For this review, take the finished solid that the model builds, in its own axes (mm). Face numbers are marked on the shaded views. A direction names the side the tool comes from. Round coordinates to 2 decimals unless told otherwise and drop trailing zeros. Order: outer loops, then holes, each group sorted by start corner. A loop starts at its lowest first (then second) coordinate and runs counter-clockwise, first axis right, second up. Notation, with made-up numbers: (57, -17) -> (78, -17) arc R25 ccw to (78, 22) -> close; hole circle Ø1 at (5.25, -11). An arc over 180 degrees is marked (long way). Use a Markdown table: item, result. Add a question column.
1) Draft analysis for pull direction Z (two halves, no side actions). For the marked faces 1, 2, 3 and 4, state which applies: pulls with the +Z half, pulls with the -Z half, needs draft (parallel to the pull), parting line crosses it, or undercut.
2) Consider section A-A (y = 0). State the section outline as (x, z) points (3 decimals).
3) Clearance check with flat-ended pins moving along their axes: P1, Ø4.5, axis at x = -0.5, y = -1, coming from the -Z side; P2, Ø3, axis at x = -4, y = 1.5, coming from the +Z side; P3, Ø0.7, axis at y = 8, z = -2.5, coming from the +X side. State where each tip first meets the part, or that it passes through.
4) Consider section C-C (z = -7.5). State the section outline as (x, y) points.
5) Consider section B-B (x = 6.75). State the section outline as (y, z) points, plus the area to 3 significant figures.
6) Machinability: for the marked faces 5, 6 and 7, which of the approach directions +Z, -Z, +X, -X, +Y, -Y give a long, thin tool a straight path to every point of the face, cutting with its end or side? Answer none if there is none.
7) Wall thickness on line 1 along Z through (x, y) = (-0.75, -6); line 2 along Y through (x, z) = (0, -26.05); line 3 along X through (y, z) = (12.75, 6.5): over which ranges is each line inside the solid? List them lowest first. Write a range as [from, to].
8) Consider section D-D (x = 0). State the section outline as (y, z) points (3 decimals), plus the area to 3 significant figures.
```python
from build123d import *

# Parameters (mm, degrees)
CROQUIS1_R              = 7.705
SALIENTE_EXTRUIR1_DEPTH = 4.35
SALIENTE_EXTRUIR2_START = -13.5
SALIENTE_EXTRUIR2_DEPTH = 18.5
SALIENTE_EXTRUIR3_DEPTH = 13.5
CROQUIS5_R              = 1.042712332
CORTAR_EXTRUIR1_DEPTH   = 2.5


with BuildPart() as part:
    # Croquis1 → Saliente-Extruir1 (new, symmetric)
    with BuildSketch(Plane.XY):
        Circle(CROQUIS1_R)
    saliente_extruir1 = extrude(amount=SALIENTE_EXTRUIR1_DEPTH, both=True)



with BuildPart() as body_2:
    # Croquis3 → Saliente-Extruir2 (new body)
    with BuildSketch(Plane.XY.offset(4.35).offset(SALIENTE_EXTRUIR2_START)):
        with BuildLine():
            Line((2, 8.034909184), (1.02204697, 8.135386739))
            ThreePointArc((1.02204697, 8.135386739), (0, 8.18775285), (-1.02204697, 8.135386739))
            Line((-1.02204697, 8.135386739), (-2, 8.034909184))
            Line((-2, 8.034909184), (-3.200003677, 11.21841322))
            ThreePointArc((-3.200003677, 11.21841322), (-3.248411026, 11.748541167), (-3.017934695, 12.228394865))
            Line((-3.017934695, 12.228394865), (-2.568482545, 12.743765532))
            ThreePointArc((-2.568482545, 12.743765532), (-2.445625709, 12.919659287), (-2.363117092, 13.117711661))
            Line((-2.363117092, 13.117711661), (-2, 14.346858197))
            Line((-2, 14.346858197), (2, 14.346858197))
            Line((2, 14.346858197), (2.363117092, 13.117711661))
            ThreePointArc((2.363117092, 13.117711661), (2.445625709, 12.919659287), (2.568482545, 12.743765532))
            Line((2.568482545, 12.743765532), (3.017934695, 12.228394865))
            ThreePointArc((3.017934695, 12.228394865), (3.248411026, 11.748541167), (3.200003677, 11.21841322))
            Line((3.200003677, 11.21841322), (2, 8.034909184))
        make_face()
    saliente_extruir2 = extrude(amount=SALIENTE_EXTRUIR2_DEPTH)


with BuildPart() as part_1:
    add(part.part)

    add(body_2.part)  # Saliente-Extruir3 merges body 2
    # Croquis4 → Saliente-Extruir3 (add)
    with BuildSketch(Plane.XY.offset(4.35)):
        with BuildLine():
            Line((1.529777798, 7.551609424), (1.529777798, 8.083221093))
            ThreePointArc((1.529777798, 8.083221093), (0, 8.18775285), (-1.529777798, 8.083221093))
            Line((-1.529777798, 8.083221093), (-1.529777798, 7.551609424))
            Line((-1.529777798, 7.551609424), (-1.529777798, 7.414435005))
            ThreePointArc((-1.529777798, 7.414435005), (0, 7.562302456), (1.529777798, 7.414435005))
            Line((1.529777798, 7.414435005), (1.529777798, 7.551609424))
        make_face()
    saliente_extruir3 = extrude(amount=-SALIENTE_EXTRUIR3_DEPTH)

    # Simetría2: Saliente-Extruir2, Saliente-Extruir3 across plane
    add(saliente_extruir2.mirror(Plane.XY.offset(-8.65)))
    add(saliente_extruir3.mirror(Plane.XY.offset(-8.65)))

    # Simetría3: Saliente-Extruir1 across plane
    add(saliente_extruir1.mirror(Plane.XY.offset(-8.65)))

    # Croquis5 → Cortar-Extruir1 (cut)
    with BuildSketch(Plane.XY.offset(9.35)):
        with Locations((0, 11.126169976)):
            Circle(CROQUIS5_R)
    cortar_extruir1 = extrude(amount=-CORTAR_EXTRUIR1_DEPTH, mode=Mode.SUBTRACT)

    # Simetría4: Cortar-Extruir1 across plane
    add(cortar_extruir1.mirror(Plane.XY.offset(-8.65)), mode=Mode.SUBTRACT)


solid = part_1.part
```
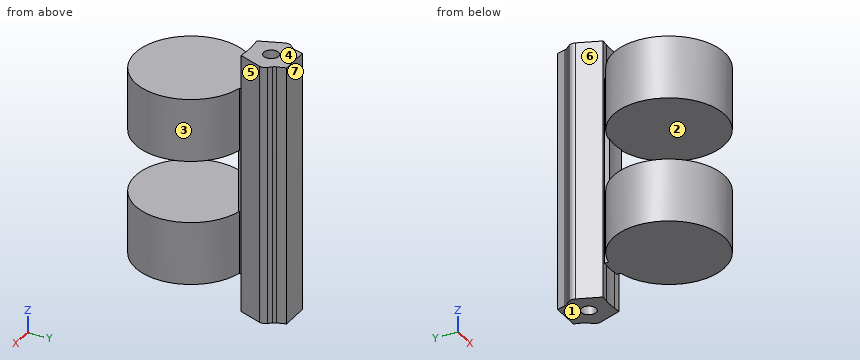
Results list:
| question | item | result |
|---|---|---|
| 1 | face 1 | pulls with the -Z half |
| 1 | face 2 | undercut |
| 1 | face 3 | needs draft |
| 1 | face 4 | pulls with the +Z half |
| 2 | outline | (-7.705, -21.65) -> (7.705, -21.65) -> (7.705, -12.95) -> (-7.705, -12.95) -> close; (-7.705, -4.35) -> (7.705, -4.35) -> (7.705, 4.35) -> (-7.705, 4.35) -> close |
| 3 | P1 | z = -21.65 |
| 3 | P2 | z = 4.35 |
| 3 | P3 | x = 2.12 |
| 4 | outline | (-3.2, 11.22) -> (-2, 8.03) -> (-1.53, 8.08) -> (-1.53, 7.41) arc R7.99 cw to (1.53, 7.41) -> (1.53, 8.08) -> (2, 8.03) -> (3.2, 11.22) arc R1 ccw to (3.02, 12.23) -> (2.57, 12.74) arc R1 cw to (2.36, 13.12) -> (2, 14.35) -> (-2, 14.35) -> (-2.36, 13.12) arc R1 cw to (-2.57, 12.74) -> (-3.02, 12.23) arc R1 ccw to start |
| 5 | outline | (-3.72, -21.65) -> (3.72, -21.65) -> (3.72, -12.95) -> (-3.72, -12.95) -> close; (-3.72, -4.35) -> (3.72, -4.35) -> (3.72, 4.35) -> (-3.72, 4.35) -> close |
| 5 | area | 129 mm2 |
| 6 | face 5 | +Z, -Z, +X |
| 6 | face 6 | +Z, -Z, -X |
| 6 | face 7 | +Z, -Z, +X, -X, +Y |
| 7 | line 1 | [-21.65, -12.95], [-4.35, 4.35] |
| 7 | line 2 | [8.19, 10.08], [12.17, 14.35] |
| 7 | line 3 | [-2.56, 2.56] |
| 8 | outline | (-7.705, -21.65) -> (8.188, -21.65) -> (8.188, -26.65) -> (10.083, -26.65) -> (10.083, -24.15) -> (12.169, -24.15) -> (12.169, -26.65) -> (14.347, -26.65) -> (14.347, 9.35) -> (12.169, 9.35) -> (12.169, 6.85) -> (10.083, 6.85) -> (10.083, 9.35) -> (8.188, 9.35) -> (8.188, 4.35) -> (-7.705, 4.35) -> (-7.705, -4.35) -> (7.562, -4.35) -> (7.562, -12.95) -> (-7.705, -12.95) -> close |
| 8 | area | 493 mm2 |
